from build123d import *

# Parameters (mm, degrees)
SKETCH1_R           = 1.27
BOSS_EXTRUDE1_DEPTH = 1.5875
FILLET1_R           = 1.27
SKETCH2_W           = 25.654
SKETCH2_H           = 30.48
BOSS_EXTRUDE2_DEPTH = 2.3749
SKETCH3_W           = 4.445
SKETCH3_H           = 6.2738
BOSS_EXTRUDE3_DEPTH = 2.8829


with BuildPart() as part:
    # Sketch1 → Boss-Extrude1 (new body)
    with BuildSketch(Plane.XY):
        Polygon((-15.24, 20.32), (15.24, 20.32), (15.24, -20.32), (10.16, -20.32), (10.16, -15.24), (-10.16, -15.24), (-10.16, -20.32), (-15.24, -20.32), align=None)
        with Locations((-12.7, -17.78)):
            Circle(SKETCH1_R, mode=Mode.SUBTRACT)
        with Locations((12.7, -17.78)):
            Circle(SKETCH1_R, mode=Mode.SUBTRACT)
        with Locations((-12.7, 17.78)):
            Circle(SKETCH1_R, mode=Mode.SUBTRACT)
        with Locations((12.7, 17.78)):
            Circle(SKETCH1_R, mode=Mode.SUBTRACT)
    extrude(amount=BOSS_EXTRUDE1_DEPTH)

    # Fillet1
    fillet1_edges = [part.edges().sort_by_distance(p)[0] for p in [
        (-15.24, 20.32, 0.79375),
        (15.24, 20.32, 0.79375),
        (15.24, -20.32, 0.79375),
        (10.16, -20.32, 0.79375),
        (-10.16, -20.32, 0.79375),
        (-15.24, -20.32, 0.79375),
    ]]
    fillet(fillet1_edges, radius=FILLET1_R)

    # Sketch2 → Boss-Extrude2 (add)
    with BuildSketch(Plane(origin=(0, 0, 0), x_dir=(-1, 0, 0), z_dir=(0, 0, -1))):
        Rectangle(SKETCH2_W, SKETCH2_H)
    extrude(amount=BOSS_EXTRUDE2_DEPTH)

    # Sketch3 → Boss-Extrude3 (add)
    with BuildSketch(Plane.XY.offset(1.5875)):
        with Locations((-12.7635, 0.0381)):
            Rectangle(SKETCH3_W, SKETCH3_H)
        with Locations((12.7635, 0.0381)):
            Rectangle(SKETCH3_W, SKETCH3_H)
    extrude(amount=BOSS_EXTRUDE3_DEPTH)


solid = part.part
Source: CAD feature listing. Evaluate the final solid. Frame: model axes, mm. A direction names the side the tool comes from. Give positions to 0.01 mm unless a question says otherwise; leave off trailing zeros. Order: outer loops, then holes, each group sorted by start corner. A loop starts at its lowest first (then second) coordinate and runs counter-clockwise, first axis right, second up. Notation, with made-up numbers: (0, 27) -> (31, 27) arc R23 cw to (31, 59) -> close; hole circle Ø4 at (-14, -36.75). An arc over 180 degrees is marked (long way). Use a Markdown table: item, result.
1) Contact query for flat-ended pins moving along their axis: P1, Ø1.9, axis at x = 3, z = -1, coming from the +Y side; P2, Ø3, axis at x = 13.5, z = 3.5, coming from the -Y side; P3, Ø0.9, axis at x = -13.5, z = 2.5, coming from the +Y side (3 decimals); P4, Ø2, axis at y = -7.5, z = 3.5, coming from the +X side. Output: stop coordinate, or through.
Answer list:
| item | result |
|---|---|
| P1 | y = 15.24 |
| P2 | y = -3.1 |
| P3 | y = 3.175 |
| P4 | through |
2) Ray query, line 1 along Y through (x, z) = (12.7, 0.7); line 2 along Z through (x, y) = (1, -9.5); line 3 along X through (y, z) = (9.5, -1.25). Return the intervals inside material, ascending. Write a range as [from, to].
Answer list:
| item | result |
|---|---|
| line 1 | [-20.32, -19.05], [-16.51, 16.51], [19.05, 20.32] |
| line 2 | [-2.37, 1.59] |
| line 3 | [-12.83, 12.83] |
3) Section query B-B, the plane z = 2. Return the cut outline in (x, y) (3 decimals), then the cut area to 3 significant figures.
Answer list:
| item | result |
|---|---|
| outline | (-14.986, -3.099) -> (-10.541, -3.099) -> (-10.541, 3.175) -> (-14.986, 3.175) -> close; (10.541, -3.099) -> (14.986, -3.099) -> (14.986, 3.175) -> (10.541, 3.175) -> close |
| area | 55.8 mm² |
4) Reachability of faces 1 (the cylindrical face through (10.542, -19.958, 0.805)), 2 (the flat face through (0, 15.24, -1)), 3 (the flat face through (14.986, 0, 3)), 4 (the flat face through (-12.827, 0, -1)), 5 (the flat face through (-13, 3.175, 3)) from +Z, -Z, +X, -X, +Y, -Y: full face, straight path, thin tool, end or side. Return the list, or none.
Answer list:
| item | result |
|---|---|
| face 1 | +Z, -Z, -Y |
| face 2 | -Z, +X, -X, +Y |
| face 3 | +Z, +X, +Y, -Y |
| face 4 | -Z, -X, +Y, -Y |
| face 5 | +Z, +X, -X, +Y |
5) Mould query, pull axis X, two halves, no side actions, for faces 6 (the flat face through (-13, 0, 4.47)), 7 (the flat face through (0, -15.24, 0)), 8 (the cylindrical face through (14.858, 19.958, 0.805)). Classes: +X half, -X half, draft (parallel to the pull), parting line (faces both ways), or undercut.
Answer list:
| item | result |
|---|---|
| face 6 | draft |
| face 7 | undercut |
| face 8 | +X half |
6) Section query A-A, the plane y = -17.78. Return the cut outline in (x, z).
Answer list:
| item | result |
|---|---|
| outline | (-15.24, 0) -> (-13.97, 0) -> (-13.97, 1.59) -> (-15.24, 1.59) -> close; (-11.43, 0) -> (-10.16, 0) -> (-10.16, 1.59) -> (-11.43, 1.59) -> close; (10.16, 0) -> (11.43, 0) -> (11.43, 1.59) -> (10.16, 1.59) -> close; (13.97, 0) -> (15.24, 0) -> (15.24, 1.59) -> (13.97, 1.59) -> close |
7) Section query D-D, the plane x = 5.5. Return the cut outline in (y, z), then the cut area to 3 significant figures.
Answer list:
| item | result |
|---|---|
| outline | (-15.24, -2.37) -> (15.24, -2.37) -> (15.24, 0) -> (20.32, 0) -> (20.32, 1.59) -> (-15.24, 1.59) -> close |
| area | 129 mm² |
8) Section query C-C, the plane y = 17.78. Return the cut outline in (x, z).
Answer list:
| item | result |
|---|---|
| outline | (-15.24, 0) -> (-13.97, 0) -> (-13.97, 1.59) -> (-15.24, 1.59) -> close; (-11.43, 0) -> (11.43, 0) -> (11.43, 1.59) -> (-11.43, 1.59) -> close; (13.97, 0) -> (15.24, 0) -> (15.24, 1.59) -> (13.97, 1.59) -> close |
